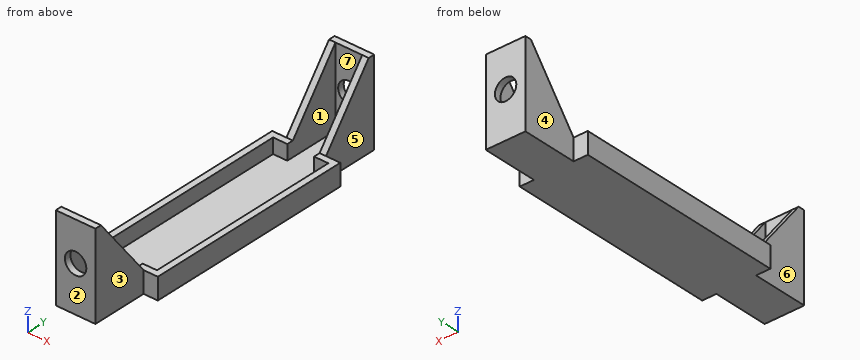
from build123d import *

# Parameters (mm, degrees)
BOSS_EXTRUDE11_DEPTH    = 40
SKETCH17_W              = 47.22521337
SKETCH17_H              = 85.181086333
CUT_EXTRUDE6_DEPTH      = 30
SHELL3_START            = -37.625
SHELL3_OUTLINE_W        = 25.8
SHELL3_OUTLINE_H        = 7
SHELL3_DEPTH            = 46.25
SHELL3_START_2          = 8.625
SHELL3_2_OUTLINE_W      = 12.5
SHELL3_2_OUTLINE_H      = 7
SHELL3_2_DEPTH          = 26
SKETCH18_W              = 54.471727392
SKETCH18_H              = 147.372956823
CUT_EXTRUDE7_DEPTH      = 308
BOSS_EXTRUDE12_DEPTH    = 3
BOSS_EXTRUDE13_DEPTH    = 2
CUT_EXTRUDE8_DEPTH      = 154.652399916
CUT_EXTRUDE8_DEPTH_BACK = 154.652399916
SKETCH21_R              = 5


# Read off the part's stored shape, not the designer's step: Shell3
with BuildPart() as part:
    # Sketch16 → Boss-Extrude11 (new body)
    with BuildSketch(Plane.XY):
        Polygon((-15.9, -37.625), (15.9, -37.625), (15.9, 11.625), (9.25, 11.625), (9.25, 37.625), (-9.25, 37.625), (-9.25, 11.625), (-15.9, 11.625), align=None)
    extrude(amount=BOSS_EXTRUDE11_DEPTH)

    # Sketch17 → Cut-Extrude6 (cut)
    with BuildSketch(Plane.XY.offset(40)):
        with Locations((3.242513711, -7.965543167)):
            Rectangle(SKETCH17_W, SKETCH17_H)
    extrude(amount=-CUT_EXTRUDE6_DEPTH, mode=Mode.SUBTRACT)

    # Shell3 outline → Shell3 (cut)
    with BuildSketch(Plane(origin=(0, 0, 0), x_dir=(1, 0, 0), z_dir=(0, 1, 0)).offset(SHELL3_START)):
        with Locations((0, -6.5)):
            Rectangle(SHELL3_OUTLINE_W, SHELL3_OUTLINE_H)
    extrude(amount=SHELL3_DEPTH, mode=Mode.SUBTRACT)

    # Shell3 2 outline → Shell3 2 (cut)
    with BuildSketch(Plane(origin=(0, 0, 0), x_dir=(1, 0, 0), z_dir=(0, 1, 0)).offset(SHELL3_START_2)):
        with Locations((0, -6.5)):
            Rectangle(SHELL3_2_OUTLINE_W, SHELL3_2_OUTLINE_H)
    extrude(amount=SHELL3_2_DEPTH, mode=Mode.SUBTRACT)

    # Sketch18 → Cut-Extrude7 (cut)
    with BuildSketch(Plane.XY.offset(40)):
        with Locations((-27.235863696, -36.061478412)):
            Rectangle(SKETCH18_W, SKETCH18_H)
    extrude(amount=-CUT_EXTRUDE7_DEPTH, mode=Mode.SUBTRACT)

    # Sketch19 → Boss-Extrude12 (add)
    with BuildSketch(Plane(origin=(9.25, 0, 0), x_dir=(0, 0, -1), z_dir=(1, 0, 0))):
        Polygon((-40, 34.625), (-10, 11.625), (-10, 34.625), align=None)
    extrude(amount=-BOSS_EXTRUDE12_DEPTH)

    # Sketch20 → Boss-Extrude13 (add)
    with BuildSketch(Plane.ZY.offset(-6.25)):
        Polygon((3, 34.625), (8, 34.625), (3, 31.625), align=None)
    extrude(amount=BOSS_EXTRUDE13_DEPTH)

    # Mirror3: part across plane


with BuildPart() as part_1:
    add(part.part)
    add(part.part.mirror(Plane(origin=(0, 37.625, -268), x_dir=(0, 0, 1), z_dir=(1, 0, 0))))

    # Mirror4: part across plane


with BuildPart() as part_2:
    add(part_1.part)
    add(part_1.part.mirror(Plane(origin=(-15.9, -37.625, 40), x_dir=(0, 0, 1), z_dir=(0, 1, 0))))

    # Sketch21 → Cut-Extrude8 (cut, two sides: drawn at the far end of the back side and taken through both)
    with BuildSketch(Plane.XZ.offset(-34.625).offset(-CUT_EXTRUDE8_DEPTH_BACK)):
        with Locations(Location((0, 21.5, 0), (0, 0, 270))):
            Circle(SKETCH21_R)
    extrude(amount=CUT_EXTRUDE8_DEPTH + CUT_EXTRUDE8_DEPTH_BACK, mode=Mode.SUBTRACT)


solid = part_2.part
Part model, mm, in its own coordinate system. Face numbers are marked on the shaded views. A direction names the side the tool comes from. Round coordinates to 2 decimals unless told otherwise and drop trailing zeros. Loops run counter-clockwise (first coordinate to the right, second up) from the corner with the lowest first, then second, coordinate; pieces in that order, holes last. Notation, with made-up numbers: (-26, -9.75) - (32, -9.75) arc R11 ccw to (32, -2.75) - close; hole circle Ø4 at (62.25, -16.5). An arc over 180 degrees is marked (long way). Answer as a JSON object with one key per item and string values.
Item 1: Pull direction Y, two halves, no side cores. Call the marked faces 1, 2 and 3: pulls with the +Y half, pulls with the -Y half, needs draft (parallel to the pull), parting line crosses it, or undercut.
Output:
{"face 1": "undercut", "face 2": "pulls with the -Y half", "face 3": "needs draft"}
Item 2: Band-saw the part on C-C on y = -45. List the corners of the cut face in (x, z).
Output:
{"outline": "(-15.9, 0) - (15.9, 0) - (15.9, 10) - (12.9, 10) - (12.9, 3) - (-12.9, 3) - (-12.9, 10) - (-15.9, 10) - close"}
Item 3: Band-saw the part on D-D on z = 21.5. List the corners of the cut face in (x, y) (3 decimals).
Output:
{"outline": "(-9.25, -112.875) - (-5, -112.875) - (-5, -109.875) - (-6.25, -109.875) - (-6.25, -95.692) - (-9.25, -95.692) - close; (-9.25, 20.442) - (-6.25, 20.442) - (-6.25, 34.625) - (-5, 34.625) - (-5, 37.625) - (-9.25, 37.625) - close; (5, -112.875) - (9.25, -112.875) - (9.25, -95.692) - (6.25, -95.692) - (6.25, -109.875) - (5, -109.875) - close; (5, 34.625) - (6.25, 34.625) - (6.25, 20.442) - (9.25, 20.442) - (9.25, 37.625) - (5, 37.625) - close"}
Item 4: Pin check, flat tips, straight feed: pin 1 (21 mm diameter, centred on y = -101.5, z = 28.5, fed in from -X); pin 2 (7.5 mm diameter, centred on x = -10.5, z = 6, fed in from -Y) (3 decimals); pin 3 (1.5 mm diameter, centred on x = -7.5, y = -87, fed in from +Z); pin 4 (3.5 mm diameter, centred on x = -13.5, z = 6.5, fed in from -Y) (3 decimals). Stop position of each tip, or through.
Output:
{"pin 1": "x = -9.25", "pin 2": "y = -112.875", "pin 3": "z = 11.14", "pin 4": "y = -86.875"}
Item 5: Band-saw the part on A-A on x = 0. List the corners of the cut face in (y, z) (3 decimals).
Output:
{"outline": "(-112.875, 0) - (37.625, 0) - (37.625, 16.5) - (34.625, 16.5) - (34.625, 3) - (-109.875, 3) - (-109.875, 16.5) - (-112.875, 16.5) - close; (-112.875, 26.5) - (-109.875, 26.5) - (-109.875, 40) - (-112.875, 40) - close; (34.625, 26.5) - (37.625, 26.5) - (37.625, 40) - (34.625, 40) - close"}
Item 6: Wall check: L1, parallel to X at y = 36.15, z = 21.5; L2, parallel to X at y = -94, z = 17; L3, parallel to Z at x = 0, y = 36. Give the ranges that are in metal, low to high.
Output:
{"L1": "-9.25 to -5, 5 to 9.25", "L2": "-9.25 to -6.25, 6.25 to 9.25", "L3": "0 to 16.5, 26.5 to 40"}
Item 7: Tool access for the marked faces 4, 5, 6 and 7: list every direction of +Z, -Z, +X, -X, +Y, -Y with a clear straight run to the whole face (end or side of a thin tool).
Output:
{"face 4": "+Z, -Z, -X, +Y", "face 5": "+Z, -Z, +X, +Y", "face 6": "+Z, -Z, -X, -Y", "face 7": "+Z"}
Item 8: Band-saw the part on B-B on z = 13. List the corners of the cut face in (x, y) (3 decimals), plus the area to 3 significant figures.
Output:
{"outline": "(-9.25, -112.875) - (9.25, -112.875) - (9.25, -89.175) - (6.25, -89.175) - (6.25, -109.875) - (-6.25, -109.875) - (-6.25, -89.175) - (-9.25, -89.175) - close; (-9.25, 13.925) - (-6.25, 13.925) - (-6.25, 34.625) - (6.25, 34.625) - (6.25, 13.925) - (9.25, 13.925) - (9.25, 37.625) - (-9.25, 37.625) - close", "area": "359 mm2"}
